Can you work these out from the model? Positions are in its coordinate system, mm. Face numbers are marked on the shaded views. A direction names the side the tool comes from. Give positions to 0.01 mm unless a question says otherwise; leave off trailing zeros. Loops run counter-clockwise (first coordinate to the right, second up) from the corner with the lowest first, then second, coordinate; pieces in that order, holes last. Notation, with made-up numbers: (32, 68) - (46, 68) arc R13 cw to (46, 73) - close; hole circle Ø3 at (48, 53.5). An arc over 180 degrees is marked (long way). Answer as a JSON object with one key per item and string values.
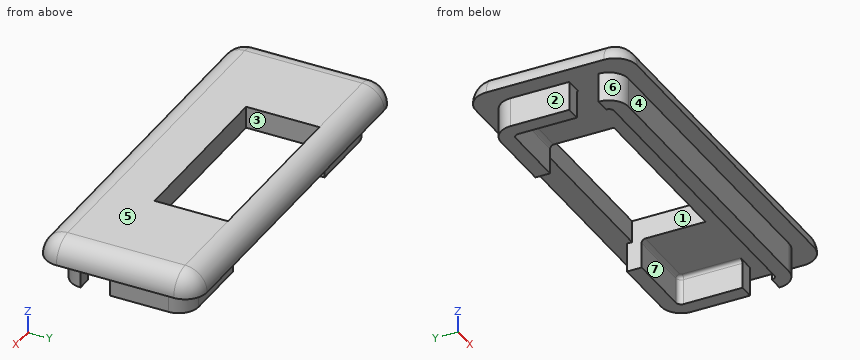
```python
from build123d import *

# Parameters (mm, degrees)
BOSS_EXTRUDE1_DEPTH   = 2
BOSS_EXTRUDE1_2_DEPTH = 2
BOSS_EXTRUDE2_DEPTH   = 1.5
FILLET1_R             = 1.5
SKETCH4_W             = 12
SKETCH4_H             = 5
CUT_EXTRUDE1_DEPTH    = 1.5
SKETCH5_W             = 12
SKETCH5_H             = 1
CUT_EXTRUDE2_DEPTH    = 2
FILLET2_R             = 0.25


with BuildPart() as part:
    # Sketch2 → Boss-Extrude1 (new body)
    with BuildSketch(Plane.XY):
        with BuildLine():
            Line((11.85, -0.425762181), (10.85, -0.425762181))
            ThreePointArc((10.85, -0.425762181), (10.747487373, -0.673249555), (10.5, -0.775762181))
            Line((10.5, -0.775762181), (-10.5, -0.775762181))
            ThreePointArc((-10.5, -0.775762181), (-10.747487373, -0.673249555), (-10.85, -0.425762181))
            Line((-10.85, -0.425762181), (-11.85, -0.425762181))
            ThreePointArc((-11.85, -0.425762181), (-11.454594155, -1.380356336), (-10.5, -1.775762181))
            Line((-10.5, -1.775762181), (10.5, -1.775762181))
            ThreePointArc((10.5, -1.775762181), (11.454594155, -1.380356336), (11.85, -0.425762181))
        make_face()
    extrude(amount=-BOSS_EXTRUDE1_DEPTH)



with BuildPart() as body_2:
    # Sketch2 → Boss-Extrude1 2 (new body)
    with BuildSketch(Plane.XY):
        with BuildLine():
            Line((11.85, 1.574237819), (10.85, 1.574237819))
            Line((10.85, 1.574237819), (10.85, 5.574237819))
            ThreePointArc((10.85, 5.574237819), (10.747487373, 5.821725192), (10.5, 5.924237819))
            Line((10.5, 5.924237819), (-10.5, 5.924237819))
            ThreePointArc((-10.5, 5.924237819), (-10.747487373, 5.821725192), (-10.85, 5.574237819))
            Line((-10.85, 5.574237819), (-10.85, 1.574237819))
            Line((-10.85, 1.574237819), (-11.85, 1.574237819))
            Line((-11.85, 1.574237819), (-11.85, 5.574237819))
            ThreePointArc((-11.85, 5.574237819), (-11.454594155, 6.528831973), (-10.5, 6.924237819))
            Line((-10.5, 6.924237819), (10.5, 6.924237819))
            ThreePointArc((10.5, 6.924237819), (11.454594155, 6.528831973), (11.85, 5.574237819))
            Line((11.85, 5.574237819), (11.85, 1.574237819))
        make_face()
    extrude(amount=-BOSS_EXTRUDE1_2_DEPTH)


with BuildPart() as part_1:
    add(part.part)

    add(body_2.part)  # Boss-Extrude2 merges body 2
    # Sketch3 → Boss-Extrude2 (add)
    with BuildSketch(Plane.XY):
        with BuildLine():
            Line((11.6095027, 8.074237819), (-11.6095027, 8.074237819))
            ThreePointArc((-11.6095027, 8.074237819), (-12.670162872, 7.63489799), (-13.1095027, 6.574237819))
            Line((-13.1095027, 6.574237819), (-13.1095027, -1.425762181))
            ThreePointArc((-13.1095027, -1.425762181), (-12.670162872, -2.486422353), (-11.6095027, -2.925762181))
            Line((-11.6095027, -2.925762181), (11.6095027, -2.925762181))
            ThreePointArc((11.6095027, -2.925762181), (12.670162872, -2.486422353), (13.1095027, -1.425762181))
            Line((13.1095027, -1.425762181), (13.1095027, 6.574237819))
            ThreePointArc((13.1095027, 6.574237819), (12.670162872, 7.63489799), (11.6095027, 8.074237819))
        make_face()
    extrude(amount=BOSS_EXTRUDE2_DEPTH)

    # Fillet1
    fillet1_edges = [part_1.edges().sort_by_distance(p)[0] for p in [
        (12.670162872, 7.63489799, 1.5),
        (13.1095027, 2.574237819, 1.5),
        (12.670162872, -2.486422353, 1.5),
        (0, -2.925762181, 1.5),
        (-12.670162872, -2.486422353, 1.5),
        (-13.1095027, 2.574237819, 1.5),
        (-12.670162872, 7.63489799, 1.5),
        (0, 8.074237819, 1.5),
    ]]
    fillet(fillet1_edges, radius=FILLET1_R - 0.0001)  # a hair under: the kernel refuses the full size

    # Sketch4 → Cut-Extrude1 (cut)
    with BuildSketch(Plane.XY.offset(1.5)):
        with Locations((0, 4.074237819)):
            Rectangle(SKETCH4_W, SKETCH4_H)
    extrude(amount=-CUT_EXTRUDE1_DEPTH, mode=Mode.SUBTRACT)

    # Sketch5 → Cut-Extrude2 (cut)
    with BuildSketch(Plane(origin=(0, 0, -2), x_dir=(-1, 0, 0), z_dir=(0, 0, -1))):
        with Locations((0, 6.424237819)):
            Rectangle(SKETCH5_W, SKETCH5_H)
    extrude(amount=-CUT_EXTRUDE2_DEPTH, mode=Mode.SUBTRACT)

    # Fillet2
    fillet2_edges = [part_1.edges().sort_by_distance(p)[0] for p in [
        (0, -0.775762181, 0),
        (10.747487373, -0.673249555, 0),
        (10.747487373, 5.821725192, 0),
        (10.85, 3.574237819, 0),
        (-10.85, 3.574237819, 0),
        (-10.747487373, 5.821725192, 0),
        (-8.25, 5.924237819, 0),
        (8.25, 5.924237819, 0),
        (-10.747487373, -0.673249555, 0),
    ]]
    fillet(fillet2_edges, radius=FILLET2_R)


solid = part_1.part
```
1) If we mould it in two halves opening along Y, with no side actions, what happens to the marked faces 1, 2, 3 and 4? For each: released by +Y, released by -Y, zero draft, split by the parting line, or undercut.
Check sheet entries:
{"face 1": "undercut", "face 2": "zero draft", "face 3": "undercut", "face 4": "released by -Y"}
2) Which directions (+Z, -Z, +X, -X, +Y, -Y) give clear straight access to the entire face, cutting with the end or side of a thin tool? Please do the marked faces 5, 6 and 7.
Check sheet entries:
{"face 5": "+Z, +X, -X, +Y, -Y", "face 6": "-Z, -X, -Y", "face 7": "-Z"}
3) Imagine slicing it at B-B on z = -0.75. Write out the boundary of the cut face in (x, y).
Check sheet entries:
{"outline": "(-11.85, -0.43) arc R1.35 ccw to (-10.5, -1.78) - (10.5, -1.78) arc R1.35 ccw to (11.85, -0.43) - (10.85, -0.43) arc R0.35 cw to (10.5, -0.78) - (-10.5, -0.78) arc R0.35 cw to (-10.85, -0.43) - close; (-11.85, 1.57) - (-10.85, 1.57) - (-10.85, 5.57) arc R0.35 cw to (-10.5, 5.92) - (-6, 5.92) - (-6, 6.92) - (-10.5, 6.92) arc R1.35 ccw to (-11.85, 5.57) - close; (6, 5.92) - (10.5, 5.92) arc R0.35 cw to (10.85, 5.57) - (10.85, 1.57) - (11.85, 1.57) - (11.85, 5.57) arc R1.35 ccw to (10.5, 6.92) - (6, 6.92) - close"}
4) I need wall thicknesses on L1, parallel to Y at x = 6.5, z = -1.9; L2, parallel to X at y = 2.25, z = -1.1. Which ranges of each line are inside material? Lowest first, please.
Check sheet entries:
{"L1": "-1.78 to -0.78, 5.92 to 6.92", "L2": "-11.85 to -10.85, 10.85 to 11.85"}
5) I'm going to push flat-ended pins straight in: P1, Ø3.5, axis at x = -3.5, y = 5, coming from the -Z side; P2, Ø0.9, axis at x = 8, z = -1.5, coming from the -Y side; P3, Ø0.5, axis at y = 3, z = -1.5, coming from the +X side. Where does each tip first touch, or does it pass through?
Check sheet entries:
{"P1": "z = 0", "P2": "y = -1.78", "P3": "x = 11.85"}
